Input: part model. Units: mm. Frame: model coordinates. A direction names the side the tool comes from. Round coordinates to 2 decimals unless told otherwise and drop trailing zeros. Answer as CSV lines item,"result". Start each with the question number.
1) Access query for faces 1 (the face through (17, -4.826, 20)), 2 (the face through (30.15, -23.44, 7.78)). Directions: +Z, -Z, +X, -X, +Y, -Y. A direction counts if a zero-diameter tool reaches every point of the face in a straight line with its end or side. Return the directions, or none.
2) Line query: L1, parallel to Y at x = 0, z = 19 (1 decimal); L2, parallel to X at y = -2.5, z = 7.5; L3, parallel to Z at x = 64, y = -2. Output: solid intervals per line, ascending.
3) First-contact query: P1, Ø3, axis at x = 18, z = 27, coming from the +Y side; P2, Ø4, axis at y = 22, z = 11, coming from the -X side; P3, Ø1.5, axis at y = -18, z = 26.5, coming from the -X side; P4, Ø17, axis at x = 0, y = 0, coming from the +Z side (3 decimals). Flat tips, straight axial feed; report the tip coordinate or a pass-through.
4) Section query B-B, the plane z = 8. State how many separate pieces and enclosed holes the cut face has, and give its area (3 significant figures).
```python
from build123d import *

# Parameters (mm, degrees)
F1_DEPTH = 40.2336
F0_R     = 10.16
F2_DEPTH = 15.7734
F3_R     = 3.302


# Not quite as in the source:
# - a feature names something its author has since deleted; it is built from what else it names


with BuildPart() as f1:
    # F0 (on Top) → F1 (new body)
    with BuildSketch(Plane.XY):
        with BuildLine():
            ThreePointArc((6.9836113022, -27.7084788139), (22.5398238454, -17.5637970274), (28.575, 0))
            ThreePointArc((28.575, 0), (22.1437005793, 18.0606519721), (5.7447533049, 27.9915779203))
            ThreePointArc((5.7447533049, 27.9915779203), (-28.5679347598, -0.6353963805), (6.9836113022, -27.7084788139))
        make_face()
        with BuildLine():
            ThreePointArc((13.4477648793, -4.826), (-14.2875, 0), (13.4477648793, 4.826))
            Line((13.4477648793, 4.826), (19.7977648793, 4.826))
            Line((19.7977648793, 4.826), (19.7977648793, -4.826))
            Line((19.7977648793, -4.826), (13.4477648793, -4.826))
        make_face(mode=Mode.SUBTRACT)
    extrude(amount=F1_DEPTH)

    # F0 (on Top) → F2 (join)
    with BuildSketch(Plane.XY):
        with BuildLine():
            ThreePointArc((5.7447533049, 27.9915779203), (22.1437005793, 18.0606519721), (28.575, 0))
            ThreePointArc((28.575, 0), (22.5398238454, -17.5637970274), (6.9836113022, -27.7084788139))
            Line((6.9836113022, -27.7084788139), (53.975, -19.05))
            ThreePointArc((53.975, -19.05), (34.925, 0), (53.975, 19.05))
            Line((53.975, 19.05), (5.7447533049, 27.9915779203))
        make_face()
        with BuildLine():
            ThreePointArc((73.025, 0), (67.4453841816, 13.4703841816), (53.975, 19.05))
            ThreePointArc((53.975, 19.05), (34.925, 0), (53.975, -19.05))
            ThreePointArc((53.975, -19.05), (67.4453841816, -13.4703841816), (73.025, 0))
        make_face()
        with Locations((53.975, 0)):
            Circle(F0_R, mode=Mode.SUBTRACT)
    extrude(amount=F2_DEPTH)

    # F3
    f3_edges = [f1.edges().sort_by_distance(p)[0] for p in [
        (-6.983611, 27.708479, 40.2336),
    ]]
    fillet(f3_edges, radius=F3_R)


solid = f1.part
```
Findings:
1,face 1,"+Z, -Z"
1,face 2,"+Z, -Z, +X, -Y"
2,L1,"y = -28.6 to -14.3, 14.3 to 28.6"
2,L2,"x = -28.47 to -14.07, 19.8 to 44.13, 63.82 to 72.86"
2,L3,"z = 0 to 15.77"
3,P1,"stops at y = 23.33"
3,P2,"stops at x = -20.41"
3,P3,"stops at x = -22.78"
3,P4,"passes through"
4,separate pieces,"1"
4,enclosed holes,"2"
4,area,"3,420 mm^2"
